For this review, take the finished solid that the model builds, in its own axes (mm). Coordinates: 2 decimals unless noted, no trailing zeros. Order: outer loops, then holes, each group sorted by start corner. A loop starts at its lowest first (then second) coordinate and runs counter-clockwise, first axis right, second up. Notation, with made-up numbers: (31.25, 17) -> (59.25, 17) arc R11 ccw to (59.25, 24) -> close; hole circle Ø2 at (-31, 53). An arc over 180 degrees is marked (long way). Return JSON: item names as keys, results as strings. Group by question number.
Item 1: Take a section at C-C (x = -6). Write out the cut boundary in (y, z).
Item 2: For line 1 along Y through (x, z) = (32, 5); line 2 along Z through (x, y) = (4, 2.5); line 3 along X through (y, z) = (1, 5.5), list the stretches that pass through material, from the lowest coordinate up.
Item 3: Insertion check: pin 1 (3.5 mm diameter, centred on y = 28, z = 11, fed in from -X); pin 2 (0.9 mm diameter, centred on y = 27, z = 11, fed in from +X); pin 3 (1 mm diameter, centred on y = 14.5, z = 8.5, fed in from -X); pin 4 (2.5 mm diameter, centred on x = 31.11, y = 12.02, fed in from +Z). Each pin has a flat end and moves straight along its axis. Give the tip position at first contact, or say it passes through.
Item 4: Take a section at D-D (y = 34). Write out the cut boundary in (x, z), then the cut area to 3 significant figures.
Item 5: Take a section at B-B (z = 3.25). Write out the cut boundary in (x, y), then the cut area to 3 significant figures.
Item 6: Take a section at A-A (x = 0). Write out the cut boundary in (y, z).
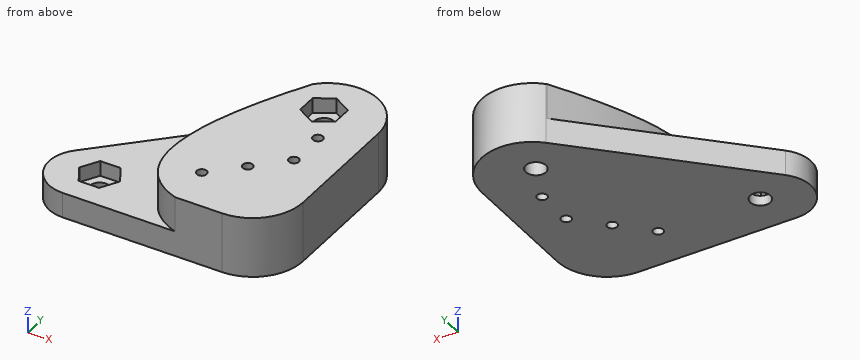
Autodesk Inventor part; units mm, degrees
ref_plane "YZ Plane" through (0, 0, 0) normal (1, 0, 0) x (0, 1, 0)
ref_plane "XZ Plane" through (0, 0, 0) normal (0, 1, 0) x (-1, 0, 0)
ref_plane "XY Plane" through (0, 0, 0) normal (0, 0, 1) x (1, 0, 0)
sketch "Esquisse1" plane through (0, 0, 0) normal (0, 0, 1) x (1, 0, 0)
  line L0 (0, 0) -> (52, 0) construction
  line L1 (0, 0) -> (25.4558, 25.4558) construction
  line L2 (0, 0) -> (-9.5459, 9.5459) construction
  line L3 (-9.5459, 9.5459) -> (-4.9497, 14.1421) construction
  line L4 (-4.9497, 14.1421) -> (0.7071, 19.799) construction
  line L5 (0.7071, 19.799) -> (6.364, 25.4558) construction
  line L6 (6.364, 25.4558) -> (12.0208, 31.1127) construction
  line L7 (25.4558, 25.4558) -> (19.799, 31.1127) construction
  line L8 (0, 0) -> (27.5772, 27.5772) construction
  circle A0 centre (0.7071, 19.799) radius 1 construction
  circle A1 centre (6.364, 25.4558) radius 1 construction
  circle A2 centre (12.0208, 31.1127) radius 1 construction
  circle A3 centre (19.799, 31.1127) radius 1 construction
  circle A4 centre (19.799, 0.7071) radius 1
  circle A5 centre (25.4558, 6.364) radius 1
  circle A6 centre (31.1127, 12.0208) radius 1
  circle A7 centre (31.1127, 19.799) radius 1
  circle A8 centre (27.5772, 27.5772) radius 2
  circle A9 centre (0, 0) radius 2
  line L9 (0, 0) -> (0, -8) construction
  line L10 (31.1127, 12.0208) -> (39.1127, 12.0208) construction
  line L11 (39.1127, 50.4264) -> (39.1127, -8)
  line L12 (0, 0) -> (-5.6569, 5.6569) construction
  line L13 (39.1127, -8) -> (-19.3137, -8)
  line L14 (-19.3137, -8) -> (39.1127, 50.4264)
  dimension "d31" = 45
  dimension "d32" = 13.5
  dimension "d33" = 6.5
  dimension "d34" = 8
  dimension "d35" = 8
  dimension "d36" = 8
  dimension "d37" = 8
  dimension "d38" = 36
  dimension "d39" = 39
  dimension "d40" = 2
  dimension "d41" = 4
  dimension "d44" = 8
  dimension "d45" = 8
  dimension "d64" = 8
extrude "Extrusion7" add sketch "Esquisse1" along normal blind 12
sketch "Esquisse7" plane through (0, 0, 12) normal (0, 0, 1) x (1, 0, 0)
  circle A0 centre (0, 0) radius 2
  circle A1 centre (27.5772, 27.5772) radius 2
  circle A2 centre (19.799, 0.7071) radius 1
  line L0 (39.1127, 50.4264) -> (-19.3137, -8)
  line L1 (-19.3137, -8) -> (39.1127, -8)
  circle A3 centre (0, 0) radius 12 construction
  circle A4 centre (19.799, 0.7071) radius 7.8116 construction
  circle A5 centre (27.5772, 27.5772) radius 8 construction
  line L2 (19.799, 0.7071) -> (19.799, -8) construction
  spline S0 degree 2 poles (19.799, -8) (2.3764, -1.7891) (21.9203, 33.234) knots 0 0 0 1 1 1
  point P0 (11.9924, 0.4283)
  dimension "d67" = 24
extrude "Extrusion8" cut sketch "Esquisse7" against normal blind 7 contours S0 L1 L0
sketch "Esquisse8" plane through (0, 0, 5) normal (0, 0, 1) x (1, 0, 0)
  circle A0 centre (0, 0) radius 2
  line L0 (19.799, -8) -> (-19.3137, -8)
  line L1 (4.0415, 0) -> (2.0207, -3.5)
  line L2 (2.0207, -3.5) -> (-2.0207, -3.5)
  line L3 (-2.0207, -3.5) -> (-4.0415, 0)
  line L4 (-4.0415, 0) -> (-2.0207, 3.5)
  line L5 (-2.0207, 3.5) -> (2.0207, 3.5)
  line L6 (2.0207, 3.5) -> (4.0415, 0)
  line L7 (2.0207, 3.5) -> (2.0207, -3.5) construction
  dimension "d70" = 7
extrude "Extrusion9" cut sketch "Esquisse8" against normal blind 3
sketch "Esquisse9" plane through (0, 0, 12) normal (0, 0, 1) x (1, 0, 0)
  line L0 (39.1127, -8) -> (39.1127, 50.4264)
  circle A0 centre (27.5772, 27.5772) radius 2
  line L1 (31.0772, 29.5979) -> (31.0772, 25.5564)
  line L2 (31.0772, 25.5564) -> (27.5772, 23.5357)
  line L3 (27.5772, 23.5357) -> (24.0772, 25.5564)
  line L4 (24.0772, 25.5564) -> (24.0772, 29.5979)
  line L5 (24.0772, 29.5979) -> (27.5772, 31.6186)
  line L6 (27.5772, 31.6186) -> (31.0772, 29.5979)
  line L7 (24.0772, 29.5979) -> (31.0772, 29.5979) construction
  point P0 (0, 0)
  dimension "d73" = 7
extrude "Extrusion10" cut sketch "Esquisse9" against normal blind 3
fillet "Congé2" radius 7 1 edges at (-19.3137, -8, 2.5)
fillet "Congé3" radius 10 1 edges at (39.1127, 50.4264, 6)
fillet "Congé4" radius 10 1 edges at (39.1127, -8, 6)
properties part number "joint1+ax12imprint"
Findings below:
{
 "1": {"outline": "(-7.01, 0) -> (5.31, 0) -> (5.31, 5) -> (-7.01, 5) -> close"},
 "2": {"line 1": "y = -7.57 to 11.56, 12.48 to 19.34, 20.26 to 35.86", "line 2": "z = 0 to 5", "line 3": "x = 11.87 to 18.84, 20.76 to 39.06"},
 "3": {"pin 1": "stops at x = 18.25", "pin 2": "stops at x = 39.11", "pin 3": "stops at x = 13.27", "pin 4": "stops at z = 12"},
 "4": {"outline": "(22.75, 0) -> (35.47, 0) -> (35.47, 12) -> (22.75, 12) -> close", "area": "153 mm2"},
 "5": {"outline": "(-7.36, 3.95) arc R7 ccw to (-2.41, -8) -> (29.11, -8) arc R10 ccw to (39.11, 2) -> (39.11, 26.28) arc R10 ccw to (22.04, 33.36) -> close; hole (-4.04, 0) -> (-2.02, -3.5) -> (2.02, -3.5) -> (4.04, 0) -> (2.02, 3.5) -> (-2.02, 3.5) -> close; hole circle Ø2 at (19.8, 0.71); hole circle Ø2 at (25.46, 6.36); hole circle Ø4 at (27.58, 27.58); hole circle Ø2 at (31.11, 12.02); hole circle Ø2 at (31.11, 19.8)", "area": "1,430 mm2"},
 "6": {"outline": "(-8, 0) -> (-2, 0) -> (-2, 2) -> (-3.5, 2) -> (-3.5, 5) -> (-8, 5) -> close; (2, 0) -> (11.31, 0) -> (11.31, 5) -> (3.5, 5) -> (3.5, 2) -> (2, 2) -> close"}
}
